Build history of the part. All positions in model axes, mm. Face numbers are marked on the shaded views. Round coordinates to 2 decimals unless told otherwise and drop trailing zeros. Write each loop counter-clockwise with the first axis right and the second up, starting at its lowest first coordinate (ties: lowest second). Pieces come first, ordered by that corner, then holes. Notation, with made-up numbers: (-37, 81.25) - (-16, 81.25) arc R34 cw to (-16, 118.25) - close; hole circle Ø5 at (46, 6). An arc over 180 degrees is marked (long way). One line per question, with ' | ' between items.
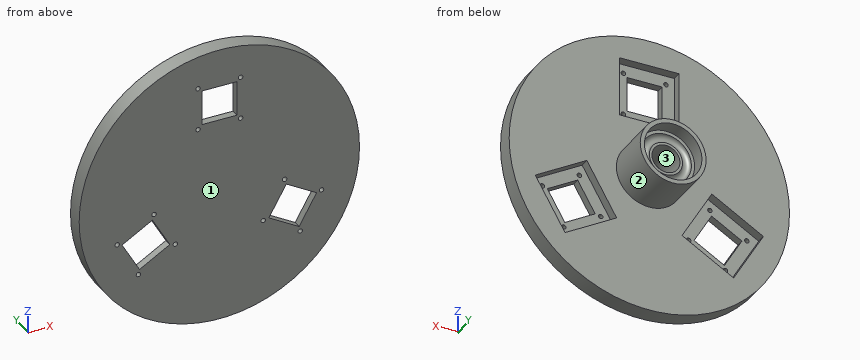
Autodesk Inventor part; units mm, degrees
ref_plane "YZ Plane" through (0, 0, 0) normal (1, 0, 0) x (0, 1, 0)
ref_plane "XZ Plane" through (0, 0, 0) normal (0, 1, 0) x (-1, 0, 0)
ref_plane "XY Plane" through (0, 0, 0) normal (0, 0, 1) x (1, 0, 0)
sketch "Sketch1" plane through (0, 0, 0) normal (0, 1, 0) x (-1, 0, 0)
  circle A0 centre (0, 0) radius 100
  dimension "d0" = 200
extrude "Extrusion1" add sketch "Sketch1" against normal blind 12
sketch "Sketch2" plane through (0, 0, 0) normal (0, 1, 0) x (1, 0, 0)
  circle A0 centre (0, 0) radius 23.5
  circle A1 centre (0, 0) radius 20.5
  dimension "d3" = 47
  dimension "d33" = 3
extrude "Extrusion2" add sketch "Sketch2" along normal blind 33
sketch "Sketch7" plane through (0, 0, 0) normal (0, 1, 0) x (1, 0, 0)
  circle A0 centre (0, 0) radius 20.5
  circle A1 centre (0, 0) radius 17.5
  circle A2 centre (0, 0) radius 10
  dimension "d37" = 35
  dimension "d40" = 20
extrude "Extrusion7" add sketch "Sketch7" along normal blind 23 contours A0 | A1
sketch "Sketch8" plane through (0, 0, 0) normal (1, 0, 0) x (0, 1, 0)
  line L0 (0, -100) -> (0, 100)
  circle A0 centre (0, 5) radius 3.175
  line L1 (-4.445, 0) -> (4.445, 0)
  point P0 (0, 0)
  point P1 (0, 0)
  dimension "d41" = 6.35
  dimension "d42" = 5
revolve "Revolution1" cut sketch "Sketch8" angle 360 about axis through (0, -10, 0) along (0, 1, 0)
sketch "Sketch9" plane through (0, 0, 0) normal (1, 0, 0) x (0, 1, 0)
  circle A0 centre (23, 15) radius 3.175
  line L0 (23, 10) -> (23, -10)
  line L1 (23, 20.5) -> (23, -20.5)
  line L2 (-5.235, 0) -> (31.41, 0)
  point P0 (0, 0)
  point P1 (23, 0)
  point P2 (23, 11.825)
  point P3 (23, 18.175)
  dimension "d44" = 6.35
  dimension "d45" = 15
revolve "Revolution2" cut sketch "Sketch9" angle 360 about axis through (0, -10, 0) along (0, 1, 0) picked at (21.9494, 14.8724) contours L1 A0
sketch "Sketch10" plane through (0, 0, 0) normal (0, 1, 0) x (1, 0, 0)
  line L0 (-15.2, -45) -> (15.2, -45) construction
  line L1 (15.2, -45) -> (15.2, -75.4) construction
  line L2 (15.2, -75.4) -> (-15.2, -75.4) construction
  line L3 (-15.2, -75.4) -> (-15.2, -45) construction
  circle A0 centre (-15.2, -45) radius 1.6
  circle A1 centre (15.2, -45) radius 1.6
  circle A2 centre (-15.2, -75.4) radius 1.6
  circle A3 centre (15.2, -75.4) radius 1.6
  point P0 (0, 0)
  point P1 (0, -45)
  point P2 (15.2, -60.2)
  dimension "d47" = 30.4
  dimension "d48" = 30.4
  dimension "d49" = 3.2
  dimension "d52" = 30.4
  dimension "d55" = 30.4
  dimension "d58" = 45
extrude "Extrusion8" cut sketch "Sketch10" against normal through all
pattern_circular "Circular Pattern2" count 3 over 360 about axis through (0, 0, 0) along (0, -1, 0) of "Extrusion8"
sketch "Sketch11" plane through (0, 0, 0) normal (0, 1, 0) x (1, 0, 0)
  line L0 (-21.25, -39.2) -> (21.25, -39.2)
  line L1 (21.25, -39.2) -> (21.25, -81.7)
  line L2 (21.25, -81.7) -> (-21.25, -81.7)
  line L3 (-21.25, -81.7) -> (-21.25, -39.2)
  point P0 (0, 0)
  point P1 (0, -39.2)
  dimension "d64" = 42.5
  dimension "d65" = 42.5
  dimension "d66" = 39.2
extrude "Extrusion9" cut sketch "Sketch11" against normal blind 6.5
pattern_circular "Circular Pattern3" count 3 over 360 about axis through (0, 0, 0) along (0, -1, 0) of "Extrusion9"
sketch "Sketch12" plane through (0, -6.5, 0) normal (0, 1, 0) x (1, 0, 0)
  line L0 (-12.5, -47.95) -> (12.5, -47.95)
  line L1 (12.5, -47.95) -> (12.5, -72.95)
  line L2 (12.5, -72.95) -> (-12.5, -72.95)
  line L3 (-12.5, -72.95) -> (-12.5, -47.95)
  line L4 (-21.25, -39.2) -> (21.25, -39.2)
  line L5 (21.25, -39.2) -> (21.25, -81.7)
  point P0 (0, 0)
  point P1 (0, -47.95)
  point P2 (0, -39.2)
  point P3 (12.5, -60.45)
  point P4 (21.25, -60.45)
  dimension "d72" = 25
  dimension "d73" = 25
extrude "Extrusion10" cut sketch "Sketch12" against normal through all
pattern_circular "Circular Pattern4" count 3 over 360 about axis through (0, 0, 0) along (0, -1, 0) of "Extrusion10"
properties part number "fixed_base"
Q1. Drop flat-ended pins along their axis: pin 1 (6 mm diameter, centred on x = 24.5, z = 38.5, fed in from +Y); pin 2 (3 mm diameter, centred on y = 0.5, z = 50, fed in from -X); pin 3 (6 mm diameter, centred on y = 16.5, z = -18.5, fed in from -X). Give the stop position or say it passes through.
Found:
pin 1: y = 0 | pin 2: x = -87.4 | pin 3: x = -17.66
Q2. Saw through at B-B, the plane x = 78.5. List the corners of the cut face in (y, z), then the cut area to 3 significant figures.
Found:
outline: (-12, -61.95) - (0, -61.95) - (0, -27.43) - (-6.5, -27.43) - (-6.5, -20.78) - (0, -20.78) - (0, 61.95) - (-12, 61.95) - close | area: 1,440 mm^2
Q3. Drill centre lines: L1, parallel to X at y = 30, z = 0; L2, parallel to Z at x = 15, y = -9; L3, parallel to X at y = 6.5, z = 0. Where is each one in solid material? Low to high. Write a range as from..to.
Found:
L1: -23.5..-20.5, 20.5..23.5 | L2: -98.87..43.41, 46.59..73.81, 76.99..98.87 | L3: -23.5..-10, 10..23.5
Q4. Saw through at A-A, the plane z = -29. List the corners of the cut face in (x, y).
Found:
outline: (-95.7, -12) - (-67.49, -12) - (-67.49, -6.5) - (-77.6, -6.5) - (-77.6, 0) - (-95.7, 0) - close; (-38.62, -12) - (38.62, -12) - (38.62, -6.5) - (28.52, -6.5) - (28.52, 0) - (-28.52, 0) - (-28.52, -6.5) - (-38.62, -6.5) - close; (67.49, -12) - (95.7, -12) - (95.7, 0) - (77.6, 0) - (77.6, -6.5) - (67.49, -6.5) - close
Q5. Pull direction X, two halves, no side cores. Call the marked faces 1, 2 and 3: +X half, -X half, draft (parallel to the pull), parting line (faces both ways), or undercut.
Found:
face 1: draft | face 2: parting line | face 3: undercut
Q6. Saw through at C-C, the plane y = 16. List the corners of the cut face in (x, z), then the cut area to 3 significant figures.
Found:
outline: circle Ø47 at (0, 0); hole circle Ø20 at (0, 0) | area: 1,420 mm^2
